```python
from build123d import *

# Parameters (mm, degrees)
SKETCH1_R                    = 1.8288
BASE_FLANGE1_DEPTH           = 1.5875
EDGE_FLANGE2_STRIP_W         = 7.8232
EDGE_FLANGE2_STRIP_H         = 1.5875
EDGE_FLANGE2_STRIP_CUT_DEPTH = 6.35
EDGE_FLANGE2_DEPTH           = 6.35
SKETCH19_W                   = 5.65
SKETCH19_H                   = 12
TAB1_DEPTH                   = 1.5875
HOLE1_START                  = -28.75
HOLE1_OUTLINE_R              = 1.8288
HOLE1_DEPTH                  = 1.5875
FILLET1_R                    = 6


# Read off the part's stored shape, not the designer's step: Hole1
# Sheet-metal steps are written as plain solids
with BuildPart() as part:
    # Sketch1 → Base-Flange1 (new body)
    with BuildSketch(Plane(origin=(0, 0, 0), x_dir=(1, 0, 0), z_dir=(0, 1, 0))):
        with BuildLine():
            Line((-25.575, 0), (-25.575, 6.35))
            Line((-25.575, 6.35), (-27.1625, 6.35))
            Line((-27.1625, 6.35), (-27.1625, 12.7))
            Line((-27.1625, 12.7), (3.175, 12.7))
            Line((3.175, 12.7), (3.175, 6.35))
            Line((3.175, 6.35), (3.175, 0))
            ThreePointArc((3.175, 0), (0, -3.175), (-3.175, 0))
            Line((-3.175, 0), (-3.175, 6.35))
            Line((-3.175, 6.35), (-19.225, 6.35))
            Line((-19.225, 6.35), (-19.225, 0))
            ThreePointArc((-19.225, 0), (-22.4, -3.175), (-25.575, 0))
        make_face()
        with Locations(Location((0, 0, 0), (0, 0, 270))):
            Circle(SKETCH1_R, mode=Mode.SUBTRACT)
        with Locations(Location((-22.4, 0, 0), (0, 0, 270))):
            Circle(SKETCH1_R, mode=Mode.SUBTRACT)
    extrude(amount=BASE_FLANGE1_DEPTH)

    # Edge-Flange2 strip (across the edge) → Edge-Flange2 strip cut (cut)
    with BuildSketch(Plane(origin=(-27.1625, 1.5875, -12.7), x_dir=(1, 0, 0), z_dir=(0, 0, 1))):
        with Locations((-3.175, -0.79375)):
            Rectangle(EDGE_FLANGE2_STRIP_W, EDGE_FLANGE2_STRIP_H)
    extrude(amount=EDGE_FLANGE2_STRIP_CUT_DEPTH, mode=Mode.SUBTRACT)

    # Edge-Flange2 section (across the edge) → Edge-Flange2 (add)
    with BuildSketch(Plane(origin=(-27.1625, 1.5875, -12.7), x_dir=(1, 0, 0), z_dir=(0, 0, 1))):
        with BuildLine():
            Line((-1.5875, 0.7366), (-1.5875, 31.688))
            Line((-1.5875, 31.688), (0, 31.688))
            Line((0, 31.688), (0, 0.7366))
            ThreePointArc((0, 0.7366), (0.215745145, 0.215745145), (0.7366, 0))
            Line((0.7366, 0), (0.7366, -1.5875))
            ThreePointArc((0.7366, -1.5875), (-0.90678687, -0.90678687), (-1.5875, 0.7366))
        make_face()
    extrude(amount=EDGE_FLANGE2_DEPTH)

    # Sketch19 → Tab1 (add)
    with BuildSketch(Plane.ZY.offset(28.75)):
        with Locations((-3.525, 27.2755)):
            Rectangle(SKETCH19_W, SKETCH19_H)
    extrude(amount=-TAB1_DEPTH)

    # Hole1 outline → Hole1 (cut)
    with BuildSketch(Plane.YZ.offset(HOLE1_START)):
        with Locations((26.9255, -6.7)):
            Circle(HOLE1_OUTLINE_R)
    extrude(amount=HOLE1_DEPTH, mode=Mode.SUBTRACT)

    # Fillet1
    # the kernel refuses this fillet: 6 mm, written as the material it takes off along each edge
    with BuildSketch(Plane(origin=(-43.724457419, 21.2755, -0.7), x_dir=(0, 0, -1), z_dir=(1, 0, 0))) as fillet1_piece_1:
        with BuildLine():
            CenterArc((6, 5.989782968), FILLET1_R, 180, 86.655847796)
            Line((0, 5.989782968), (-0.12, 5.989782968))
            Line((-0.12, 5.989782968), (-0.12, 0))
            Line((-0.12, 0), (0, -0.12))
            ThreePointArc((0, -0.12), (2.825, -0.12), (5.643, -0.119795659))
            Line((5.643, -0.119795659), (5.65, 0))
        make_face()
    extrude(amount=31.536414838, mode=Mode.SUBTRACT)
    with BuildSketch(Plane(origin=(-43.75, 33.2755, -0.7), x_dir=(0, 0, -1), z_dir=(1, 0, 0)), Plane(origin=(-43.75, 33.2755, -12.7), x_dir=(0, -1, 0), z_dir=(1, 0, 0))) as fillet1_piece_2:
        with BuildLine():
            CenterArc((FILLET1_R, -FILLET1_R), FILLET1_R, 90, 90)
            Line((0, -FILLET1_R), (-FILLET1_R * 0.02, -FILLET1_R))
            Line((-FILLET1_R * 0.02, -FILLET1_R), (-FILLET1_R * 0.02, FILLET1_R * 0.02))
            Line((-FILLET1_R * 0.02, FILLET1_R * 0.02), (FILLET1_R, FILLET1_R * 0.02))
            Line((FILLET1_R, FILLET1_R * 0.02), (FILLET1_R, 0))
        make_face()
    extrude(amount=31.5875, mode=Mode.SUBTRACT)


solid = part.part
```
Geometry: final body of the model. Coordinates: model frame, mm. A direction names the side the tool comes from. Round coordinates to 2 decimals unless told otherwise and drop trailing zeros. Write each loop counter-clockwise with the first axis right and the second up, starting at its lowest first coordinate (ties: lowest second). Pieces come first, ordered by that corner, then holes.
Item 1: Section query D-D (y = 18.5). Return loops of the section in (x, z), plus the area to 3 significant figures.
Item 2: Mould query, pull axis X, two halves, no side actions, for faces 1 (the face through (-11, 1, -6.35)), 2 (the face through (-11, 0, -7)), 3 (the face through (-28.05, 0.66, -9.57)). Classes: +X half, -X half, draft (parallel to the pull), parting line (faces both ways), or undercut.
Item 3: Set-up query: faces 4 (the face through (-19.225, 1, -3)), 5 (the face through (-17, 1, -12.7)), 6 (the face through (-27.162, 18, -8)), 7 (the face through (-25.575, 1, -3)), 8 (the face through (-28, 11, -6.35)). Return all of +Z, -Z, +X, -X, +Y, -Y with unobstructed straight access to the full face (end or side cutting, diameter ignored); none if empty.
Item 4: Material intervals for L1, parallel to X at y = 2.5, z = -9.25; L2, parallel to Y at x = -1, z = -6, sorted ascending.
Item 5: Section query A-A (x = -22.4). Return loops of the section in (y, z) (1 decimal).
Item 6: Pin query (flat end, axial travel): P1, Ø1.3, axis at x = -15, y = 1, coming from the +Z side; P2, Ø4, axis at y = 26.93, z = -6.7, coming from the +X side; P3, Ø1.3, axis at y = 0.5, z = -2, coming from the -X side (3 decimals); P4, Ø5, axis at x = -22.5, y = 11, coming from the -Z side. Return the tip coordinate at first contact, or that it passes through.
Item 7: Section query C-C (z = -5.5). Give the number of separate pieces and of enclosed holes in the cut face, plus the area to 3 significant figures.
Completed:
1. outline: (-28.75, -12.7) - (-27.16, -12.7) - (-27.16, -6.35) - (-28.75, -6.35) - close
1. area: 10.1 mm2
2. face 1: undercut
2. face 2: draft
2. face 3: -X half
3. face 4: +Z, +Y, -Y
3. face 5: -Z, +X, -X, +Y, -Y
3. face 6: +Z, -Z, +X, +Y
3. face 7: +Z, -X, +Y, -Y
3. face 8: +Z, -X, -Y
4. L1: x = -28.75 to -27.16
4. L2: y = 0 to 1.59
5. outline: (0, -12.7) - (1.6, -12.7) - (1.6, -1.8) - (0, -1.8) - close; (0, 1.8) - (1.6, 1.8) - (1.6, 3.2) - (0, 3.2) - close
6. P1: stops at z = -6.35
6. P2: stops at x = -27.16
6. P3: stops at x = -25.575
6. P4: passes through
7. separate pieces: 4
7. enclosed holes: 0
7. area: 34.5 mm2
